Verification items for the finished model (mm, model axes). Face numbers are marked on the shaded views. Round coordinates to 2 decimals unless told otherwise and drop trailing zeros. Write each loop counter-clockwise with the first axis right and the second up, starting at its lowest first coordinate (ties: lowest second). Pieces come first, ordered by that corner, then holes. Notation, with made-up numbers: (45, 24.5) - (56, 24.5) arc R17 ccw to (56, 51.5) - close; hole circle Ø6 at (88.25, -25). An arc over 180 degrees is marked (long way). Answer as a JSON object with one key per item and string values.
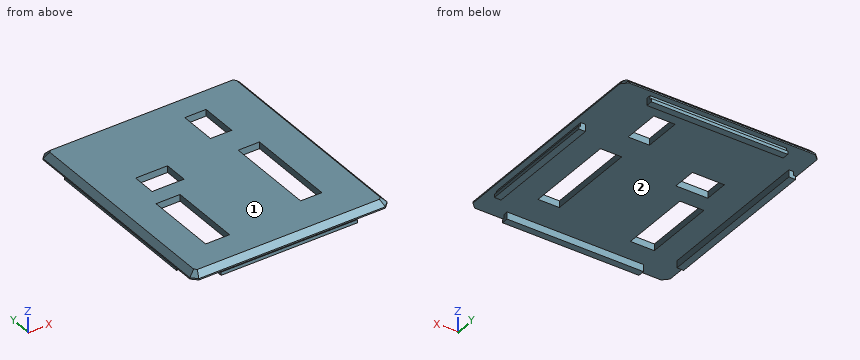
```python
from build123d import *

# Parameters (mm, degrees)
PAD006_DEPTH    = 2.5
CHAMFER001_SIZE = 2
SKETCH006_W     = 8
SKETCH006_H     = 14
SKETCH006_H_2   = 34
SKETCH006_W_2   = 9
SKETCH006_H_3   = 27
POCKET001_DEPTH = 5
SKETCH008_W     = 51.2
SKETCH008_H     = 1.8
SKETCH008_W_2   = 1.8
SKETCH008_H_2   = 46
SKETCH008_H_3   = 61
PAD007_DEPTH    = 2.65
SKETCH009_W     = 51.2
SKETCH009_H     = 0.7
SKETCH009_W_2   = 0.7
SKETCH009_H_2   = 46
SKETCH009_H_3   = 61
PAD008_DEPTH    = 1.2
SKETCH014_W     = 12
SKETCH014_H     = 9
POCKET004_DEPTH = 5


with BuildPart() as part:
    # Sketch004 → Pad006 (new body)
    with BuildSketch(Plane.XY.offset(21)):
        Polygon((-34.986794, 50.683687), (35.013206, 50.683687), (37.013212, 48.683681), (37.013212, -31.316319), (35.013206, -33.316325), (-34.986794, -33.316325), (-36.9868, -31.316319), (-36.9868, 48.683681), align=None)
    extrude(amount=PAD006_DEPTH)

    # Chamfer001
    chamfer001_edges = [part.edges().sort_by_distance(p)[0] for p in [
        (0.013206, -33.316325, 23.5),
        (-36.9868, 8.683681, 23.5),
        (-35.986797, 49.683684, 23.5),
        (0.013206, 50.683687, 23.5),
        (36.013209, 49.683684, 23.5),
        (37.013212, 8.683681, 23.5),
        (36.013209, -32.316322, 23.5),
        (-35.986797, -32.316322, 23.5),
    ]]
    chamfer(chamfer001_edges, length=CHAMFER001_SIZE)

    # Sketch006 → Pocket001 (cut)
    with BuildSketch(Plane.XY.offset(23.5)):
        with Locations((14.226603, 32.961599)):
            Rectangle(SKETCH006_W, SKETCH006_H)
        with Locations((17.619118, -1.209573)):
            Rectangle(SKETCH006_W, SKETCH006_H_2)
        with Locations((-19.565168, -7.664242)):
            Rectangle(SKETCH006_W_2, SKETCH006_H_3)
    extrude(amount=-POCKET001_DEPTH, mode=Mode.SUBTRACT)

    # Sketch008 → Pad007 (new body)
    with BuildSketch(Plane(origin=(0, 0, 21), x_dir=(1, 0, 0), z_dir=(0, 0, -1))):
        with Locations((-0.047285, 30.276958)):
            Rectangle(SKETCH008_W, SKETCH008_H)
        with Locations((33.924806, -1.191265)):
            Rectangle(SKETCH008_W_2, SKETCH008_H_2)
        with Locations((0.001681, -47.694109)):
            Rectangle(SKETCH008_W, SKETCH008_H)
        with Locations((-33.880968, -8.711103)):
            Rectangle(SKETCH008_W_2, SKETCH008_H_3)
    extrude(amount=PAD007_DEPTH)

    # Sketch009 → Pad008 (new body)
    with BuildSketch(Plane(origin=(0, 0, 18.35), x_dir=(1, 0, 0), z_dir=(0, 0, -1))):
        with Locations((-0.047285, 31.526958)):
            Rectangle(SKETCH009_W, SKETCH009_H)
        with Locations((35.174806, -1.191265)):
            Rectangle(SKETCH009_W_2, SKETCH009_H_2)
        with Locations((0.001681, -48.944109)):
            Rectangle(SKETCH009_W, SKETCH009_H)
        with Locations((-35.130968, -8.711103)):
            Rectangle(SKETCH009_W_2, SKETCH009_H_3)
    extrude(amount=-PAD008_DEPTH)

    # Sketch014 → Pocket004 (cut)
    with BuildSketch(Plane.XY.offset(23.5)):
        with Locations((-15.238739, 16.5837)):
            Rectangle(SKETCH014_W, SKETCH014_H)
    extrude(amount=-POCKET004_DEPTH, mode=Mode.SUBTRACT)


solid = part.part
```
Q1. Section check A-A, the plane y = -16.5. Record the cut outline in (x, z), then the cut area to 3 significant figures.
Geometry check:
{"outline": "(-36.99, 21) - (-34.78, 21) - (-34.78, 19.55) - (-35.48, 19.55) - (-35.48, 18.35) - (-32.98, 18.35) - (-32.98, 21) - (-24.07, 21) - (-24.07, 23.5) - (-34.99, 23.5) - (-36.99, 21.5) - close; (-15.07, 21) - (13.62, 21) - (13.62, 23.5) - (-15.07, 23.5) - close; (21.62, 21) - (33.02, 21) - (33.02, 18.35) - (35.52, 18.35) - (35.52, 19.55) - (34.82, 19.55) - (34.82, 21) - (37.01, 21) - (37.01, 21.5) - (35.01, 23.5) - (21.62, 23.5) - close", "area": "150 mm2"}
Q2. Section check D-D, the plane z = 22.55. Record the cut outline in (x, y), then the cut area to 3 significant figures.
Geometry check:
{"outline": "(-35.94, -30.88) - (-34.55, -32.27) - (34.58, -32.27) - (35.96, -30.88) - (35.96, 48.25) - (34.58, 49.63) - (-34.55, 49.63) - (-35.94, 48.25) - close; hole (-24.07, -21.16) - (-15.07, -21.16) - (-15.07, 5.84) - (-24.07, 5.84) - close; hole (-21.24, 12.08) - (-9.24, 12.08) - (-9.24, 21.08) - (-21.24, 21.08) - close; hole (10.23, 25.96) - (18.23, 25.96) - (18.23, 39.96) - (10.23, 39.96) - close; hole (13.62, -18.21) - (21.62, -18.21) - (21.62, 15.79) - (13.62, 15.79) - close", "area": "5,150 mm2"}
Q3. Material ranges on line 1 along X through (y, z) = (1, 21.25); line 2 along X through (y, z) = (-10, 20.9); line 3 along Y through (x, z) = (21, 20.7), recorded low to high. Write a range as [from, to].
Geometry check:
{"line 1": "x = [-36.99, -24.07], [-15.07, 13.62], [21.62, 37.01]", "line 2": "x = [-34.78, -32.98], [33.02, 34.82]", "line 3": "y = [-31.18, -29.38], [46.79, 48.59]"}
Q4. Section check C-C, the plane y = 35. Record the cut outline in (x, z).
Geometry check:
{"outline": "(-36.99, 21) - (-34.78, 21) - (-34.78, 19.55) - (-35.48, 19.55) - (-35.48, 18.35) - (-32.98, 18.35) - (-32.98, 21) - (10.23, 21) - (10.23, 23.5) - (-34.99, 23.5) - (-36.99, 21.5) - close; (18.23, 21) - (37.01, 21) - (37.01, 21.5) - (35.01, 23.5) - (18.23, 23.5) - close"}
Q5. Gauge pin test, flat ends, axial feed: P1, Ø1, axis at y = -21, z = 19, coming from the +X side; P2, Ø0.8, axis at y = 48, z = 19.5, coming from the -X side; P3, Ø1.2, axis at y = -4, z = 22.5, coming from the -X side. Record the tip position at first contact, or that the pin passes through.
Geometry check:
{"P1": "stops at x = 35.52", "P2": "stops at x = -25.6", "P3": "stops at x = -36.59"}
Q6. Section check B-B, the plane x = -17. Record the cut outline in (y, z), then the cut area to 3 significant figures.
Geometry check:
{"outline": "(-33.32, 21) - (-31.18, 21) - (-31.18, 19.55) - (-31.88, 19.55) - (-31.88, 18.35) - (-29.38, 18.35) - (-29.38, 21) - (-21.16, 21) - (-21.16, 23.5) - (-31.32, 23.5) - (-33.32, 21.5) - close; (5.84, 21) - (12.08, 21) - (12.08, 23.5) - (5.84, 23.5) - close; (21.08, 21) - (46.79, 21) - (46.79, 18.35) - (49.29, 18.35) - (49.29, 19.55) - (48.59, 19.55) - (48.59, 21) - (50.68, 21) - (50.68, 21.5) - (48.68, 23.5) - (21.08, 23.5) - close", "area": "127 mm2"}
Q7. Release check for a two-part mould opening along Y. For the marked faces 1 and 2 record: released by +Y, released by -Y, zero draft, split by the parting line, or undercut.
Geometry check:
{"face 1": "zero draft", "face 2": "undercut"}
